Geometry: final body of the model. Coordinates: model frame, mm. Face numbers are marked on the shaded views. A direction names the side the tool comes from. Give positions to 0.01 mm unless a question says otherwise; leave off trailing zeros. Write each loop counter-clockwise with the first axis right and the second up, starting at its lowest first coordinate (ties: lowest second). Pieces come first, ordered by that corner, then holes. Notation, with made-up numbers: (62, 78) -> (113, 78) arc R31 ccw to (113, 113) -> close; hole circle Ø1 at (27.5, 60.5). An arc over 180 degrees is marked (long way). Answer as a JSON object with one key per item and string values. Group by question number.
(1) Contact query for flat-ended pins moving along their axis: pin 1 Ø1.5 at (x, z) = (33.5, 4) entering from +Y; pin 2 Ø1.9 at (y, z) = (-2, -19.5) entering from -X; pin 3 Ø3 at (y, z) = (-4.5, 10) entering from -X; pin 4 Ø1.9 at (x, y) = (27.5, -2) entering from +Z. Output: stop coordinate, or through.
(2) Set-up query: the marked faces 4 and 5. Return all of +Z, -Z, +X, -X, +Y, -Y with unobstructed straight access to the full face (end or side cutting, diameter ignored); none if empty.
(3) Draft query along X for the marked faces 1, 2 and 3. Return one class per face: +X half, -X half, draft (parallel to the pull), parting line (faces both ways), or undercut.
(4) Material intervals for probe 1 along Z at (x, y) = (49, -1.75); probe 2 along Z at (x, y) = (-1, -3.5); probe 3 along Z at (x, y) = (37.5, -4.25), sorted ascending.
(5) Section query D-D on y = -2.5. Output: boundary loops of the cut face in (x, z).
(6) Section query C-C on z = -25. Output: boundary loops of the cut face in (x, y), plus the area to 3 significant figures.
(7) Section query A-A on z = 2. Output: boundary loops of the cut face in (x, y), plus the area to 3 significant figures.
(8) Section query B-B on x = -17.78. Output: boundary loops of the cut face in (y, z), plus the area to 3 significant figures.
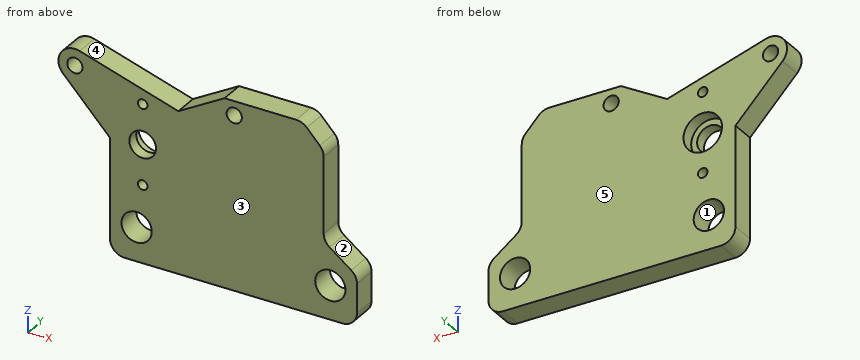
from build123d import *

# Parameters (mm, degrees)
SKETCH4_R           = 2
SKETCH4_R_2         = 1.25
SKETCH4_R_3         = 5.05
SKETCH4_R_4         = 3.96875
BOSS_EXTRUDE2_DEPTH = 6.35
SKETCH31_R          = 6.35
SKETCH31_R_2        = 3.499999985
BOSS_EXTRUDE5_DEPTH = 3


with BuildPart() as part:
    # Sketch4 → Boss-Extrude2 (new body)
    # profile 1 of 2: a face of its own
    with BuildSketch(Plane(origin=(0, 0, 0), x_dir=(1, 0, 0), z_dir=(0, 1, 0))):
        with BuildLine():
            Line((21.46596982, -18.4375), (40.257702493, -18.4375))
            ThreePointArc((40.257702493, -18.4375), (41.776936446, -18.121498883), (43.044160097, -17.225913752))
            Line((43.044160097, -17.225913752), (46.444939319, -13.579024524))
            ThreePointArc((46.444939319, -13.579024524), (47.203372649, -12.376980446), (47.468481715, -10.980610773))
            Line((47.468481715, -10.980610773), (47.468481715, 8.985116992))
            ThreePointArc((47.468481715, 8.985116992), (47.868781798, 10.685130659), (48.985566477, 12.027918285))
            Line((48.985566477, 12.027918285), (54.680415238, 16.319294633))
            ThreePointArc((54.680415238, 16.319294633), (55.797199918, 17.662082259), (56.1975, 19.362095927))
            Line((56.1975, 19.362095927), (56.1975, 26.9875))
            ThreePointArc((56.1975, 26.9875), (55.081576836, 29.681576836), (52.3875, 30.7975))
            Line((52.3875, 30.7975), (-4.7625, 30.7975))
            ThreePointArc((-4.7625, 30.7975), (-7.456576836, 29.681576836), (-8.5725, 26.9875))
            Line((-8.5725, 26.9875), (-8.5725, 0.781747009))
            Line((-8.5725, 0.781747009), (-20.917416467, -12.27322702))
            ThreePointArc((-20.917416467, -12.27322702), (-21.4498857, -17.515316011), (-16.517810325, -19.369406885))
            Line((-16.517810325, -19.369406885), (9.346561417, -11.463733294))
            Line((9.346561417, -11.463733294), (21.46596982, -18.4375))
        make_face()
        with Locations(Location((-17.78, -15.24, 0), (0, 0, 270))):
            Circle(SKETCH4_R, mode=Mode.SUBTRACT)
        with Locations(Location((0, -10.5, 0), (0, 0, 270))):
            Circle(SKETCH4_R_2, mode=Mode.SUBTRACT)
        with Locations(Location((0, 0, 0), (0, 0, 270))):
            Circle(SKETCH4_R_3, mode=Mode.SUBTRACT)
        with Locations(Location((24.012521227, -14.703599027, 0), (0, 0, 270))):
            Circle(SKETCH4_R, mode=Mode.SUBTRACT)
        with Locations(Location((0, 10.5, 0), (0, 0, 270))):
            Circle(SKETCH4_R_2, mode=Mode.SUBTRACT)
        with Locations(Location((-1.5875, 21.9075, 0), (0, 0, 270))):
            Circle(SKETCH4_R_4, mode=Mode.SUBTRACT)
        with Locations(Location((49.2125, 21.9075, 0), (0, 0, 270))):
            Circle(SKETCH4_R_4, mode=Mode.SUBTRACT)
    # profile 2 of 2: a face of its own
    with BuildSketch(Plane(origin=(0, 0, 0), x_dir=(1, 0, 0), z_dir=(0, 1, 0))):
        with BuildLine():
            Line((21.46596982, -18.4375), (40.257702493, -18.4375))
            ThreePointArc((40.257702493, -18.4375), (41.776936446, -18.121498883), (43.044160097, -17.225913752))
            Line((43.044160097, -17.225913752), (46.444939319, -13.579024524))
            ThreePointArc((46.444939319, -13.579024524), (47.203372649, -12.376980446), (47.468481715, -10.980610773))
            Line((47.468481715, -10.980610773), (47.468481715, 8.985116992))
            ThreePointArc((47.468481715, 8.985116992), (47.868781798, 10.685130659), (48.985566477, 12.027918285))
            Line((48.985566477, 12.027918285), (54.680415238, 16.319294633))
            ThreePointArc((54.680415238, 16.319294633), (55.797199918, 17.662082259), (56.1975, 19.362095927))
            Line((56.1975, 19.362095927), (56.1975, 26.9875))
            ThreePointArc((56.1975, 26.9875), (55.081576836, 29.681576836), (52.3875, 30.7975))
            Line((52.3875, 30.7975), (-4.7625, 30.7975))
            ThreePointArc((-4.7625, 30.7975), (-7.456576836, 29.681576836), (-8.5725, 26.9875))
            Line((-8.5725, 26.9875), (-8.5725, 0.781747009))
            Line((-8.5725, 0.781747009), (-20.917416467, -12.27322702))
            ThreePointArc((-20.917416467, -12.27322702), (-21.4498857, -17.515316011), (-16.517810325, -19.369406885))
            Line((-16.517810325, -19.369406885), (9.346561417, -11.463733294))
            Line((9.346561417, -11.463733294), (21.46596982, -18.4375))
        make_face()
        with Locations(Location((-17.78, -15.24, 0), (0, 0, 270))):
            Circle(SKETCH4_R, mode=Mode.SUBTRACT)
        with Locations(Location((0, -10.5, 0), (0, 0, 270))):
            Circle(SKETCH4_R_2, mode=Mode.SUBTRACT)
        with Locations(Location((0, 0, 0), (0, 0, 270))):
            Circle(SKETCH4_R_3, mode=Mode.SUBTRACT)
        with Locations(Location((24.012521227, -14.703599027, 0), (0, 0, 270))):
            Circle(SKETCH4_R, mode=Mode.SUBTRACT)
        with Locations(Location((0, 10.5, 0), (0, 0, 270))):
            Circle(SKETCH4_R_2, mode=Mode.SUBTRACT)
        with Locations(Location((-1.5875, 21.9075, 0), (0, 0, 270))):
            Circle(SKETCH4_R_4, mode=Mode.SUBTRACT)
        with Locations(Location((49.2125, 21.9075, 0), (0, 0, 270))):
            Circle(SKETCH4_R_4, mode=Mode.SUBTRACT)
    extrude(amount=-BOSS_EXTRUDE2_DEPTH)

    # Sketch31 → Boss-Extrude5 (add)
    with BuildSketch(Plane.XZ.offset(6.35)):
        Circle(SKETCH31_R)
        with Locations(Location((0, 0, 0), (0, 0, 270))):
            Circle(SKETCH31_R_2, mode=Mode.SUBTRACT)
    extrude(amount=-BOSS_EXTRUDE5_DEPTH)


solid = part.part
Answer list:
{
 "1": {"pin 1": "y = 0", "pin 2": "x = -8.57", "pin 3": "x = -20.19", "pin 4": "z = 18.44"},
 "2": {"face 4": "+Z, +Y, -Y", "face 5": "+Z, -Z, +X, -X, +Y"},
 "3": {"face 1": "undercut", "face 2": "+X half", "face 3": "draft"},
 "4": {"probe 1": "-30.8 to -25.87, -17.94 to -12.04", "probe 2": "-30.8 to -25.83, -17.98 to -11.25, -9.75 to -3.35, 3.35 to 9.75, 11.25 to 14.63", "probe 3": "-30.8 to 18.44"},
 "5": {"outline": "(-20.92, 12.27) -> (-8.57, -0.78) -> (-8.57, -26.99) arc R3.81 ccw to (-4.76, -30.8) -> (52.39, -30.8) arc R3.81 ccw to (56.2, -26.99) -> (56.2, -19.36) arc R3.81 ccw to (54.68, -16.32) -> (48.99, -12.03) arc R3.81 cw to (47.47, -8.99) -> (47.47, 10.98) arc R3.81 ccw to (46.44, 13.58) -> (43.04, 17.23) arc R3.81 ccw to (40.26, 18.44) -> (21.47, 18.44) -> (9.35, 11.46) -> (-16.52, 19.37) arc R4.32 ccw to start; hole circle Ø4 at (-17.78, 15.24); hole circle Ø7.94 at (-1.59, -21.91); hole circle Ø10.1 at (0, 0); hole circle Ø2.5 at (0, -10.5); hole circle Ø2.5 at (0, 10.5); hole circle Ø4 at (24.01, 14.7); hole circle Ø7.94 at (49.21, -21.91)"},
 "6": {"outline": "(-8.57, -6.35) -> (-4.07, -6.35) -> (-4.07, 0) -> (-8.57, 0) -> close; (0.9, -6.35) -> (46.73, -6.35) -> (46.73, 0) -> (0.9, 0) -> close; (51.7, -6.35) -> (56.2, -6.35) -> (56.2, 0) -> (51.7, 0) -> close", "area": "348 mm2"},
 "7": {"outline": "(-11.2, -6.35) -> (-2.87, -6.35) -> (-2.87, -3.35) -> (-4.64, -3.35) -> (-4.64, 0) -> (-11.2, 0) -> close; (2.87, -6.35) -> (47.47, -6.35) -> (47.47, 0) -> (4.64, 0) -> (4.64, -3.35) -> (2.87, -3.35) -> close", "area": "324 mm2"},
 "8": {"outline": "(-6.35, 8.96) -> (0, 8.96) -> (0, 13.24) -> (-6.35, 13.24) -> close; (-6.35, 17.24) -> (0, 17.24) -> (0, 19.56) -> (-6.35, 19.56) -> close", "area": "41.9 mm2"}
}
